from build123d import *

# Parameters (mm, degrees)
F1_DEPTH = 25


with BuildPart() as f1:
    # F0 (on Top) → F1 (new body)
    with BuildSketch(Plane.XY):
        with BuildLine():
            ThreePointArc((-49.834719, -13.743161), (-44.834719, -8.331543), (-39.834719, -13.743161))
            Line((-39.834719, -13.743161), (-19.834719, -13.743161))
            Line((-19.834719, -13.743161), (-19.834719, -28.743161))
            Line((-19.834719, -28.743161), (-39.834719, -28.743161))
            Line((-39.834719, -28.743161), (-39.834719, -31.743161))
            Line((-39.834719, -31.743161), (-19.971046, -31.743161))
            Line((-19.971046, -31.743161), (-16.971046, -31.743161))
            Line((-16.971046, -31.743161), (-16.971046, -11.743161))
            Line((-16.971046, -11.743161), (-55.198664, 1.256839))
            Line((-55.198664, 1.256839), (-55.198664, -13.743161))
            Line((-55.198664, -13.743161), (-49.834719, -13.743161))
        make_face()
    extrude(amount=F1_DEPTH)


solid = f1.part
Build history of the part. All positions in model axes, mm. A direction names the side the tool comes from. Give positions to 0.01 mm unless a question says otherwise; leave off trailing zeros. Order: outer loops, then holes, each group sorted by start corner. A loop starts at its lowest first (then second) coordinate and runs counter-clockwise, first axis right, second up. Notation, with made-up numbers: M 44,47.25 L 80,47.25 A9 ccw 80,56.25 Z; hole C 52.25,-28.75 d9. An arc over 180 degrees is marked long. Use one line per item in the form item = value.
1) Saw through at D-D (y = -29.5). Give the cut face in (x, z), plus the area to 3 significant figures.
Calculated:
outline = M -39.83,0 L -16.97,0 L -16.97,25 L -39.83,25 Z
area = 572 mm2
2) Saw through at B-B (y = -10.5). Give the cut face in (x, z).
Calculated:
outline = M -55.2,0 L -48.96,0 L -48.96,25 L -55.2,25 Z; M -40.71,0 L -20.63,0 L -20.63,25 L -40.71,25 Z
3) Drop flat-ended pins along their axis: pin 1 (1.6 mm diameter, centred on x = -52, z = 17, fed in from -Y); pin 2 (4.5 mm diameter, centred on y = -23.5, z = 10.5, fed in from -X); pin 3 (10 mm diameter, centred on x = -27, z = 7.5, fed in from +Y). Give the stop position or say it passes through.
Calculated:
pin_1 = -13.74
pin_2 = -19.83
pin_3 = -6.63
4) Tool access for faces 1 (the face through (-39.835, -30, 12)), 2 (the face through (-55.199, -6, 12)), 3 (the face through (-30, -13.743, 12)): list every direction of +Z, -Z, +X, -X, +Y, -Y with a clear straight run to the whole face (end or side of a thin tool).
Calculated:
face_1 = +Z, -Z, -X, -Y
face_2 = +Z, -Z, -X, +Y, -Y
face_3 = +Z, -Z, -X
5) Probe probe 1 along X at (y, z) = (-16, 4); probe 2 along X at (y, z) = (-13, 2.75); probe 3 along Y at (x, z) = (-22.5, 13.25). List the from-to ranges inside material, lowest first.
Calculated:
probe_1 = -19.83 to -16.97
probe_2 = -55.2 to -49.84, -39.83 to -16.97
probe_3 = -31.74 to -28.74, -13.74 to -9.86
6) Saw through at C-C (z = 22). Give the cut face in (x, y), plus the area to 3 significant figures.
Calculated:
outline = M -55.2,-13.74 L -49.83,-13.74 A5.02 cw long -39.83,-13.74 L -19.83,-13.74 L -19.83,-28.74 L -39.83,-28.74 L -39.83,-31.74 L -16.97,-31.74 L -16.97,-11.74 L -55.2,1.26 Z
area = 393 mm2
7) Saw through at A-A (x = -22). Give the cut face in (y, z), plus the area to 3 significant figures.
Calculated:
outline = M -31.74,0 L -28.74,0 L -28.74,25 L -31.74,25 Z; M -13.74,0 L -10.03,0 L -10.03,25 L -13.74,25 Z
area = 168 mm2
